The listing builds one solid part. Answer for the finished solid, in the listing's coordinates (mm). Round coordinates to 2 decimals unless told otherwise and drop trailing zeros. Write each loop counter-clockwise with the first axis right and the second up, starting at its lowest first coordinate (ties: lowest second). Pieces come first, ordered by that corner, then holes.
(1) Find the intervals of material crossed by probe 1 along Y at (x, z) = (4.75, 1.65) (3 decimals); probe 2 along Y at (x, z) = (-25.25, 1.9) (3 decimals); probe 3 along X at (y, z) = (28, 1.65), in increasing order.
(2) A cutting plane is placed at D-D, the plane x = 4.75. Give the vertices of the cut face in (y, z) (3 decimals), and give its area (3 significant figures).
(3) Each of these flat-tipped pins is pushed along its axis until it touches: pin 1 Ø0.9 at (y, z) = (-24.5, 2) entering from -X; pin 2 Ø0.9 at (x, z) = (-6.5, 1) entering from +Y (3 decimals); pin 3 Ø1.5 at (x, z) = (-25, 1) entering from -Y (3 decimals); pin 4 Ø2 at (x, y) = (-20, 28.395) entering from -Z. Where does it stop, or does it pass through?
(4) A cutting plane is placed at C-C, the plane y = 25.5. Give the vertices of the cut face in (x, z), and give its area (3 significant figures).
(5) A cutting plane is placed at A-A, the plane y = -15. Give the vertices of the cut face in (x, z), and give its area (3 significant figures).
(6) A cutting plane is placed at B-B, the plane x = 20. Give the vertices of the cut face in (y, z) (3 decimals).
from build123d import *

# Parameters (mm, degrees)
SKETCH1_W           = 45.5
SKETCH1_H           = 63.15
BOSS_EXTRUDE1_DEPTH = 3
SKETCH2_R           = 1.75
CUT_EXTRUDE1_DEPTH  = 3
SKETCH3_W           = 33
SKETCH3_H           = 9
CUT_EXTRUDE2_DEPTH  = 3
SKETCH4_W           = 5.5
SKETCH4_H           = 35.99
BOSS_EXTRUDE2_DEPTH = 3
SKETCH5_R           = 1.5
CUT_EXTRUDE3_DEPTH  = 3
CUT_EXTRUDE4_DEPTH  = 10


with BuildPart() as part:
    # Sketch1 → Boss-Extrude1 (new body)
    with BuildSketch(Plane.XY):
        Rectangle(SKETCH1_W, SKETCH1_H)
    extrude(amount=BOSS_EXTRUDE1_DEPTH)

    # Sketch2 → Cut-Extrude1 (cut)
    with BuildSketch(Plane.XY.offset(3)):
        with Locations((20, -28.395)):
            Circle(SKETCH2_R)
        with Locations(Location((20, 28.395, 0), (0, 0, 180))):
            Circle(SKETCH2_R)
        with Locations((-20, 28.395)):
            Circle(SKETCH2_R)
        with Locations(Location((-20, -28.395, 0), (0, 0, 180))):
            Circle(SKETCH2_R)
    extrude(amount=-CUT_EXTRUDE1_DEPTH, mode=Mode.SUBTRACT)

    # Sketch3 → Cut-Extrude2 (cut)
    with BuildSketch(Plane.XY.offset(3)):
        with Locations((-0.75, 27.075)):
            Rectangle(SKETCH3_W, SKETCH3_H)
        with Locations((-0.75, -27.075)):
            Rectangle(SKETCH3_W, SKETCH3_H)
    extrude(amount=-CUT_EXTRUDE2_DEPTH, mode=Mode.SUBTRACT)

    # Sketch4 → Boss-Extrude2 (add)
    with BuildSketch(Plane.XY.offset(3)):
        with Locations((-25.5, 0)):
            Rectangle(SKETCH4_W, SKETCH4_H)
    extrude(amount=-BOSS_EXTRUDE2_DEPTH)

    # Sketch5 → Cut-Extrude3 (cut)
    with BuildSketch(Plane(origin=(0, 0, 0), x_dir=(-1, 0, 0), z_dir=(0, 0, -1))):
        with Locations((-4.75, 15)):
            Circle(SKETCH5_R)
        with Locations((25.25, 15)):
            Circle(SKETCH5_R)
        with Locations((25.25, -15)):
            Circle(SKETCH5_R)
        with Locations((-4.75, -15)):
            Circle(SKETCH5_R)
    extrude(amount=-CUT_EXTRUDE3_DEPTH, mode=Mode.SUBTRACT)

    # Sketch6 → Cut-Extrude4 (cut)
    with BuildSketch(Plane(origin=(0, 0, 0), x_dir=(-1, 0, 0), z_dir=(0, 0, -1))):
        Polygon((-22.75, 0), (-22.75, -8.5), (-13.75, -8.5), (-13.75, 8.5), (-22.75, 8.5), align=None)
    extrude(amount=-CUT_EXTRUDE4_DEPTH, mode=Mode.SUBTRACT)


solid = part.part
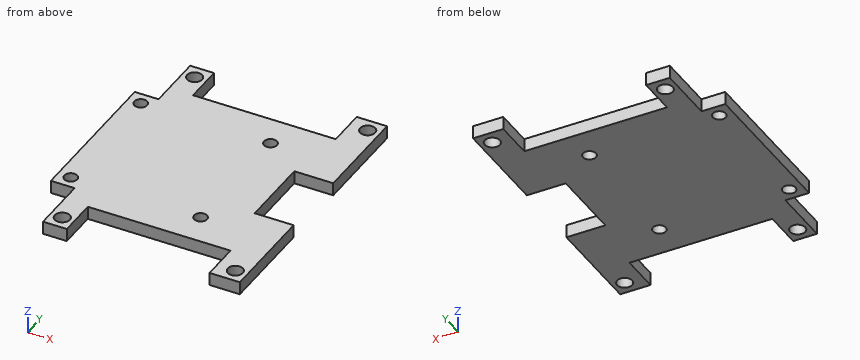
Solutions:
1. probe 1: y = -22.575 to -16.5, -13.5 to 13.5, 16.5 to 22.575
1. probe 2: y = -17.995 to -16.5, -13.5 to 13.5, 16.5 to 17.995
1. probe 3: x = -22.75 to -21.7, -18.3 to -17.25, 15.75 to 18.3, 21.7 to 22.75
2. outline: (-22.575, 0) - (-16.5, 0) - (-16.5, 3) - (-22.575, 3) - close; (-13.5, 0) - (13.5, 0) - (13.5, 3) - (-13.5, 3) - close; (16.5, 0) - (22.575, 0) - (22.575, 3) - (16.5, 3) - close
2. area: 117 mm2
3. pin 1: stops at x = -22.75
3. pin 2: stops at y = 22.575
3. pin 3: stops at y = -17.995
3. pin 4: passes through
4. outline: (-22.75, 0) - (-17.25, 0) - (-17.25, 3) - (-22.75, 3) - close; (15.75, 0) - (22.75, 0) - (22.75, 3) - (15.75, 3) - close
4. area: 37.5 mm2
5. outline: (-28.25, 0) - (-26.75, 0) - (-26.75, 3) - (-28.25, 3) - close; (-23.75, 0) - (3.25, 0) - (3.25, 3) - (-23.75, 3) - close; (6.25, 0) - (22.75, 0) - (22.75, 3) - (6.25, 3) - close
5. area: 135 mm2
6. outline: (-31.575, 0) - (-30.145, 0) - (-30.145, 3) - (-31.575, 3) - close; (-26.645, 0) - (-8.5, 0) - (-8.5, 3) - (-26.645, 3) - close; (8.5, 0) - (26.645, 0) - (26.645, 3) - (8.5, 3) - close; (30.145, 0) - (31.575, 0) - (31.575, 3) - (30.145, 3) - close
